from build123d import *

# Parameters (mm, degrees)
F0_R     = 4.7625
F0_R_2   = 1.6256
F1_DEPTH = 1.5875
F2_DEPTH = 6.35


with BuildPart() as f1:
    # F0 (on Front) → F1 (new body)
    with BuildSketch(Plane.XZ):
        Circle(F0_R)
        with BuildLine():
            ThreePointArc((-1.5702184362, -2.55625), (-1.464469988, 2.6182680639), (3, 0))
            ThreePointArc((3, 0), (2.6182680639, -1.464469988), (1.5702184362, -2.55625))
            ThreePointArc((1.5702184362, -2.55625), (0, -3), (-1.5702184362, -2.55625))
        make_face(mode=Mode.SUBTRACT)
        with BuildLine():
            ThreePointArc((1.5702184362, -2.55625), (2.6182680639, -1.464469988), (3, 0))
            ThreePointArc((3, 0), (-1.464469988, 2.6182680639), (-1.5702184362, -2.55625))
            Line((-1.5702184362, -2.55625), (0, -2.55625))
            Line((0, -2.55625), (1.5702184362, -2.55625))
        make_face()
        Circle(F0_R_2, mode=Mode.SUBTRACT)
        with BuildLine():
            Line((0, -2.55625), (-1.5702184362, -2.55625))
            ThreePointArc((-1.5702184362, -2.55625), (0, -3), (1.5702184362, -2.55625))
            Line((1.5702184362, -2.55625), (0, -2.55625))
        make_face()
    extrude(amount=-F1_DEPTH)

    # F0 (on Front) → F2 (join)
    with BuildSketch(Plane.XZ):
        with BuildLine():
            ThreePointArc((1.5702184362, -2.55625), (2.6182680639, -1.464469988), (3, 0))
            ThreePointArc((3, 0), (-1.464469988, 2.6182680639), (-1.5702184362, -2.55625))
            Line((-1.5702184362, -2.55625), (0, -2.55625))
            Line((0, -2.55625), (1.5702184362, -2.55625))
        make_face()
        Circle(F0_R_2, mode=Mode.SUBTRACT)
    extrude(amount=-F2_DEPTH)


solid = f1.part
Geometry: final body of the model. Coordinates: model frame, mm. A direction names the side the tool comes from. Round coordinates to 2 decimals unless told otherwise and drop trailing zeros. Loops run counter-clockwise (first coordinate to the right, second up) from the corner with the lowest first, then second, coordinate; pieces in that order, holes last.
Q1. Section C-C on y = 4.5. Return loops of the section in (x, z).
Q2. Section B-B on z = -0.25. Return loops of the section in (x, y).
Q3. Material intervals for L1, parallel to Z at x = 0, y = 3.5; L2, parallel to Z at x = 0.5, y = 4.5; L3, parallel to X at y = 1, z = -1.25, sorted ascending.
Q4. Section D-D on x = -2. Return loops of the section in (y, z), plus the area to 3 significant figures.
Q5. Pull-direction query (Z, two-part tool) for faces 3 (the cylindrical face through (-3.78, 0.78, -2.9)), 4 (the flat face through (-1, 6.35, -2)), 5 (the cylindrical face through (-0.21, 3.13, 1.61)), 6 (the flat face through (0, 4, -2.556)); classes: released by +Z, released by -Z, zero draft, split by the parting line, or undercut.
Q6. Pin query (flat end, axial travel): P1, Ø1, axis at x = -1, z = 3.5, coming from the +Y side; P2, Ø3, axis at x = -3, y = 4, coming from the -Z side; P3, Ø1.5, axis at x = -2.5, y = 1.5, coming from the +Z side. Return the tip coordinate at first contact, or that it passes through.
Q7. Section A-A on x = 0. Return loops of the section in (y, z), plus the area to 3 significant figures.
Q8. Access query for faces 1 (the flat face through (2, 0, 0)), 2 (the flat face through (0, 1.588, -3)). Directions: +Z, -Z, +X, -X, +Y, -Y. A direction counts if a zero-diameter tool reaches every point of the face in a straight line with its end or side. Return the directions, or none.
Evaluation:
1. outline: (-1.57, -2.56) - (1.57, -2.56) arc R3 ccw (long way) to start; hole circle Ø3.25 at (0, 0)
2. outline: (-4.76, 0) - (-1.61, 0) - (-1.61, 6.35) - (-2.99, 6.35) - (-2.99, 1.59) - (-4.76, 1.59) - close; (1.61, 0) - (4.76, 0) - (4.76, 1.59) - (2.99, 1.59) - (2.99, 6.35) - (1.61, 6.35) - close
3. L1: z = -2.56 to -1.63, 1.63 to 3
3. L2: z = -2.56 to -1.55, 1.55 to 2.96
3. L3: x = -4.6 to -1.04, 1.04 to 4.6
4. outline: (0, -4.32) - (1.59, -4.32) - (1.59, -2.24) - (6.35, -2.24) - (6.35, 2.24) - (1.59, 2.24) - (1.59, 4.32) - (0, 4.32) - close
4. area: 35.0 mm2
5. face 3: split by the parting line
5. face 4: zero draft
5. face 5: undercut
5. face 6: released by -Z
6. P1: stops at y = 1.59
6. P2: stops at z = -2.56
6. P3: stops at z = 4.43
7. outline: (0, -4.76) - (1.59, -4.76) - (1.59, -2.56) - (6.35, -2.56) - (6.35, -1.63) - (0, -1.63) - close; (0, 1.63) - (6.35, 1.63) - (6.35, 3) - (1.59, 3) - (1.59, 4.76) - (0, 4.76) - close
7. area: 20.9 mm2
8. face 1: +Z, -Z, +X, -X, -Y
8. face 2: +Y
